Check sheet for the modelled part. Datum: model origin and axes. Units: mm. A direction names the side the tool comes from. Coordinates: 2 decimals unless noted, no trailing zeros. Write each loop counter-clockwise with the first axis right and the second up, starting at its lowest first coordinate (ties: lowest second). Pieces come first, ordered by that corner, then holes. Notation, with made-up numbers: (80, 12.5) -> (85, 12.5) arc R16 cw to (85, 26.5) -> close; hole circle Ø11 at (64.5, 36.5). An arc over 180 degrees is marked (long way). Put each result on its own line as item: value.
```python
from build123d import *

# Parameters (mm, degrees)
F0_R     = 355.6
F1_DEPTH = 127
F3_DEPTH = 101.6


with BuildPart() as f1:
    # F0 (on Top) → F1 (new body)
    with BuildSketch(Plane.XY):
        Circle(F0_R)
    extrude(amount=F1_DEPTH)

    # F2 (on face) → F3 (cut)
    with BuildSketch(Plane.XY.offset(127)):
        with BuildLine():
            ThreePointArc((353.0999389591, 42.0926728434), (231.1027319808, 270.2644765244), (-13.2445388494, 355.353263937))
            Line((-13.2445388494, 355.353263937), (15.4660869459, 13.7182963842))
            Line((15.4660869459, 13.7182963842), (353.0999389591, 42.0926728434))
        make_face()
        with BuildLine():
            Line((-9.9109431068, 11.5856387734), (-38.6445388494, 353.4939315139))
            ThreePointArc((-38.6445388494, 353.4939315139), (-274.5766604834, 225.962425013), (-354.3236766316, -30.1013650562))
            Line((-354.3236766316, -30.1013650562), (-8.8475509302, -1.0679325675))
            Line((-8.8475509302, -1.0679325675), (-9.9109431068, 11.5856387734))
        make_face()
        with BuildLine():
            Line((33.6104931009, -354.0080433458), (4.9256574214, -12.679958877))
            Line((4.9256574214, -12.679958877), (-7.7819411742, -13.7478914444))
            Line((-7.7819411742, -13.7478914444), (-353.0195925051, -42.7612828101))
            ThreePointArc((-353.0195925051, -42.7612828101), (-222.9891918492, -276.9967153568), (33.6104931009, -354.0080433458))
        make_face()
        with BuildLine():
            Line((355.2049530963, 16.7571267176), (17.5950888785, -11.6152338337))
            Line((17.5950888785, -11.6152338337), (46.2493560151, -352.5795755119))
            ThreePointArc((46.2493560152, -352.5795755119), (267.2991124181, -234.5262128217), (355.6, 0))
            ThreePointArc((355.6, 0), (355.5012245556, 8.3808913292), (355.2049530963, 16.7571267176))
        make_face()
    extrude(amount=-F3_DEPTH, mode=Mode.SUBTRACT)


solid = f1.part
```
Q1. Cross-section at B-B (y = -259). Record the cut outline in (x, z), plus the area to 3 significant figures.
Recorded:
outline: (-243.66, 0) -> (243.66, 0) -> (243.66, 25.4) -> (38.39, 25.4) -> (38.39, 127) -> (25.63, 127) -> (25.63, 25.4) -> (-243.66, 25.4) -> close
area: 13,700 mm2
Q2. Cross-section at A-A (z = 34.5). Record the cut outline in (x, y).
Recorded:
outline: (-354.32, -30.1) arc R355.6 ccw to (-353.02, -42.76) -> (4.93, -12.68) -> (33.61, -354.01) arc R355.6 ccw to (46.25, -352.58) -> (17.6, -11.62) -> (355.2, 16.76) arc R355.6 ccw to (353.1, 42.09) -> (15.47, 13.72) -> (-13.24, 355.35) arc R355.6 ccw to (-38.64, 353.49) -> (-8.85, -1.07) -> close
Q3. Material ranges on line 1 along Z through (x, y) = (22.5, 83); line 2 along X through (y, z) = (132, 87.5); line 3 along X through (y, z) = (-218, 83), recorded low to high.
Recorded:
line 1: z = 0 to 25.4
line 2: x = -20.03 to 5.53
line 3: x = 22.18 to 34.94
Q4. Mould release check, pull along X, two halves, no side actions. Record for faces 3 (the flat face through (25, 2, 127)), 4 (the cylindrical face through (353.763, 36.1, 20.87)), 5 (the flat face through (181.92, 27.707, 76.911)): released by +X, released by -X, zero draft, split by the parting line, or undercut.
Recorded:
face 3: zero draft
face 4: split by the parting line
face 5: undercut
Q5. Depth check by flat-ended pin: P1, Ø2, axis at y = -161.5, z = 104, coming from the +X side; P2, Ø10, axis at y = 57, z = 72.5, coming from the +X side; P3, Ø2, axis at x = 99, y = 154.5, coming from the +Z side. Enter the tip coordinate at first touch or a pass-through.
Recorded:
P1: stops at x = 30.28
P2: stops at x = 12.25
P3: stops at z = 25.4
Q6. Tool access check on faces 1 (the flat face through (31.72, -179.71, 76.91)), 2 (the flat face through (-5, 5, 0)). Record the directions out of +Z, -Z, +X, -X, +Y, -Y that give a thin tool (end or side, any length) a straight path to the whole face; none if there is none.
Recorded:
face 1: +Z, +X
face 2: -Z, +X, -X, +Y, -Y
Q7. Cross-section at C-C (x = 210). Record the cut outline in (y, z), plus the area to 3 significant figures.
Recorded:
outline: (-286.97, 0) -> (286.97, 0) -> (286.97, 25.4) -> (30.07, 25.4) -> (30.07, 127) -> (4.55, 127) -> (4.55, 25.4) -> (-286.97, 25.4) -> close
area: 17,200 mm2
